Study the drawing (mm; zero at the part's minimum x, y, z) and answer. Round coordinates to 2 decimals unless told otherwise and drop trailing zeros. Write each loop counter-clockwise with the first axis right and the second up, starting at its lowest first coordinate (ties: lowest second). Pieces come first, ordered by that corner, then holes. Notation, with made-up numbers: (9, 49) -> (68, 49) arc R18 ccw to (68, 64) -> close; hole circle Ø3 at (-9, 83.25). An arc over 180 degrees is marked (long way). Write each question's results on one line, items separated by ' | '. Start each with the question number.
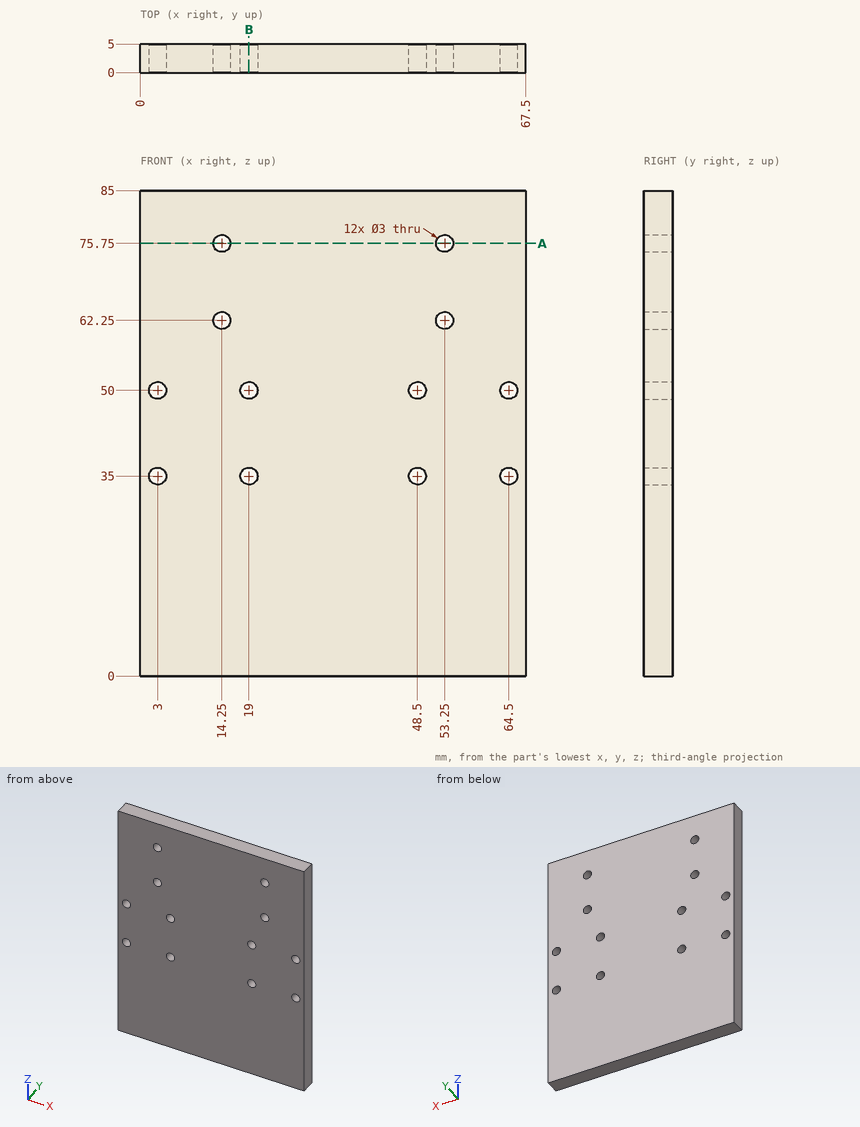
Q1. The part is cut by section B-B, the plane x = 19. Write down the section's boundary in (y, z).
Q2. This flat-tipped pin is pushed along its axis until it touches: pin 1 (1.8 mm diameter, centred on x = 64.5, z = 35, fed in from +Y). Where does it stop, or does it pass through?
Q3. Find the intervals of material crossed by line 1 (Z direction, x = 3, y = 4.3); line 2 (Z direction, x = 53.25, y = 2.75); line 3 (X direction, y = 3.85, z = 50), in increasing order.
Q4. The part is cut by section A-A, the plane z = 75.75. Write down the section's boundary in (x, y), then the cut area to 4 significant figures.
Answers follow:
1) outline: (0, 0) -> (5, 0) -> (5, 33.5) -> (0, 33.5) -> close; (0, 36.5) -> (5, 36.5) -> (5, 48.5) -> (0, 48.5) -> close; (0, 51.5) -> (5, 51.5) -> (5, 85) -> (0, 85) -> close
2) pin 1: through
3) line 1: 0 to 33.5, 36.5 to 48.5, 51.5 to 85 | line 2: 0 to 60.75, 63.75 to 74.25, 77.25 to 85 | line 3: 0 to 1.5, 4.5 to 17.5, 20.5 to 47, 50 to 63, 66 to 67.5
4) outline: (0, 0) -> (12.75, 0) -> (12.75, 5) -> (0, 5) -> close; (15.75, 0) -> (51.75, 0) -> (51.75, 5) -> (15.75, 5) -> close; (54.75, 0) -> (67.5, 0) -> (67.5, 5) -> (54.75, 5) -> close | area: 307.5 mm^2
